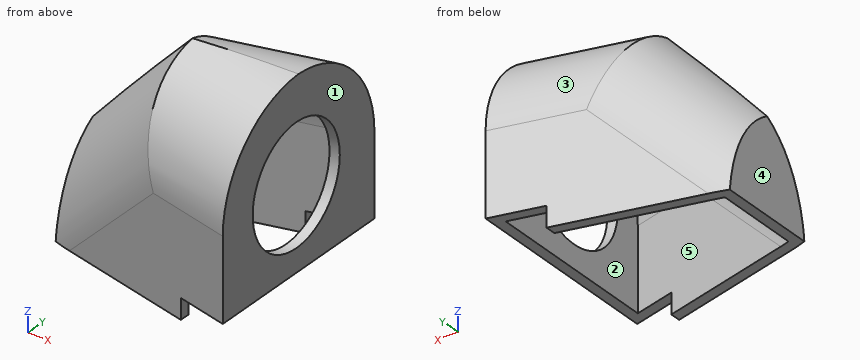
from build123d import *

# Parameters (mm, degrees)
F1_DEPTH    = 40
F2_SIZE     = 20
F3_T1_DEPTH = 120.6155281281
F3_T3_DEPTH = 120.6155281281
F3_T5_DEPTH = 112.8188914216
F3_T7_DEPTH = 112.8188914216
F5_T        = -2
F4_R        = 11.5
F6_DEPTH    = 5
F8_DEPTH    = 4


# Not quite as in the source:
# - a fillet or chamfer that OpenCascade refuses, or shapes differently, is made with other operations: its cross-section is extruded or revolved along the edge and cut away or added


with BuildPart() as f1:
    # F0 (on Top) → F1 (new body)
    with BuildSketch(Plane.XY):
        Polygon((-40, 10), (0, 0), (0, 40), (-40, 30), align=None)
    extrude(amount=F1_DEPTH)

    # F2
    f2_edges = [f1.edges().sort_by_distance(p)[0] for p in [
        (-40, 20, 40),
    ]]
    chamfer(f2_edges, length=F2_SIZE)

    # F3: fillet of radius 20 on 4 edges, made by hand

    # F3_s2 → F3_t1 (cut)
    with BuildSketch(Plane(origin=(57.9188897131, 14.4797224283, 0), x_dir=(0, 0, 1), z_dir=(-0.9701425001, -0.242535625, 0))):
        with BuildLine():
            ThreePointArc((40, 18.8057000058), (34.1421356237, 32.9478356295), (20, 38.8057000058))
            Line((20, 38.8057000058), (40, 38.8057000058))
            Line((40, 38.8057000058), (40, 18.8057000058))
        make_face()
    extrude(amount=F3_T1_DEPTH, mode=Mode.SUBTRACT)

    # F3_s4 → F3_t3 (cut)
    with BuildSketch(Plane(origin=(-68.5071250073, 17.1267812518, 0), x_dir=(0, 0, 1), z_dir=(0.9701425001, -0.242535625, 0))):
        with BuildLine():
            ThreePointArc((20, 0), (34.1421356237, -5.8578643763), (40, -20))
            Line((40, -20), (40, 0))
            Line((40, 0), (20, 0))
        make_face()
    extrude(amount=F3_T3_DEPTH, mode=Mode.SUBTRACT)

    # F3_s6 → F3_t5 (cut)
    with BuildSketch(Plane(origin=(-40.1875872415, 10.0468968104, -40.1875872415), x_dir=(0.242535625, 0.9701425001, 0), z_dir=(0.6963106238, -0.174077656, 0.6963106238))):
        with BuildLine():
            ThreePointArc((0, 26.2452181161), (4.6931480366, 39.1176803115), (16.5700282971, 45.948905439))
            Line((16.5700282971, 45.948905439), (0, 43.0644337539))
            Line((0, 43.0644337539), (0, 26.2452181161))
        make_face()
    extrude(amount=F3_T5_DEPTH, mode=Mode.SUBTRACT)

    # F3_s8 → F3_t7 (cut)
    with BuildSketch(Plane(origin=(-35.339102393, -8.8347755983, -35.339102393), x_dir=(-0.242535625, 0.9701425001, 0), z_dir=(0.6963106238, 0.174077656, 0.6963106238))):
        with BuildLine():
            ThreePointArc((22.2356717087, 39.1937001443), (34.1125519692, 32.3624750168), (38.8057000058, 19.4900128214))
            Line((38.8057000058, 19.4900128214), (38.8057000058, 36.3092284592))
            Line((38.8057000058, 36.3092284592), (22.2356717087, 39.1937001443))
        make_face()
    extrude(amount=F3_T7_DEPTH, mode=Mode.SUBTRACT)

    # F5
    f5_openings = [f1.faces().sort_by_distance(p)[0] for p in [
        (-17.771277, 20, 0),
    ]]
    offset(amount=F5_T, openings=f5_openings)

    # F4 (on face) → F6 (cut)
    with BuildSketch(Plane.YZ):
        with Locations((19.3844718719, 20)):
            Circle(F4_R)
    extrude(amount=-F6_DEPTH, mode=Mode.SUBTRACT)

    # F7 (on face) → F8 (cut)
    with BuildSketch(Plane.XY):
        Polygon((-10.0002693493, 2.5000673373), (0, 0), (0, 40), (-10.0040400222, 37.4989899944), align=None)
    extrude(amount=F8_DEPTH, mode=Mode.SUBTRACT)


solid = f1.part
Here's how the part is built. I have some questions about the finished solid (model axes, mm). Face numbers are marked on the shaded views. A direction names the side the tool comes from. Coordinates: 2 decimals unless noted, no trailing zeros.
1. I need wall thicknesses on L1, parallel to X at y = 16, z = 9.5; L2, parallel to X at y = 32, z = 22; L3, parallel to Y at x = -16, z = 21. Which ranges of each line are inside material? Lowest first, please.
2. If we mould it in two halves opening along X, with no side actions, what happens to the marked faces 1, 2 and 3? For each: pulls with the +X half, pulls with the -X half, needs draft (parallel to the pull), parting line crosses it, or undercut.
3. For the marked faces 4 and 5, which set-ups out of +Z, -Z, +X, -X, +Y, -Y let a thin tool reach every point of the face, with its end or its side?
4. For P1, Ø20.5, axis at y = 19.38, z = 20, coming from the +X side; P2, Ø3, axis at x = -15.5, y = 32, coming from the +Z side; P3, Ø1, axis at y = 4, z = 2, coming from the +X side; P4, Ø10, axis at x = -35.5, z = 31.5, coming from the -Y side, each with a flat end and sliding along its axis, tell me the tip position at first contact or that it passes through.
Taken from the geometry:
1. L1: x = -40 to -38
1. L2: x = -25.23 to -20.85, -2 to 0
1. L3: y = 4.03 to 6.09, 33.91 to 35.97
2. face 1: pulls with the +X half
2. face 2: undercut
2. face 3: pulls with the -X half
3. face 4: +Z, -Z, -X, +Y, -Y
3. face 5: -Z
4. P1: stops at x = -23.16
4. P2: stops at z = 33.78
4. P3: stops at x = -10
4. P4: passes through
